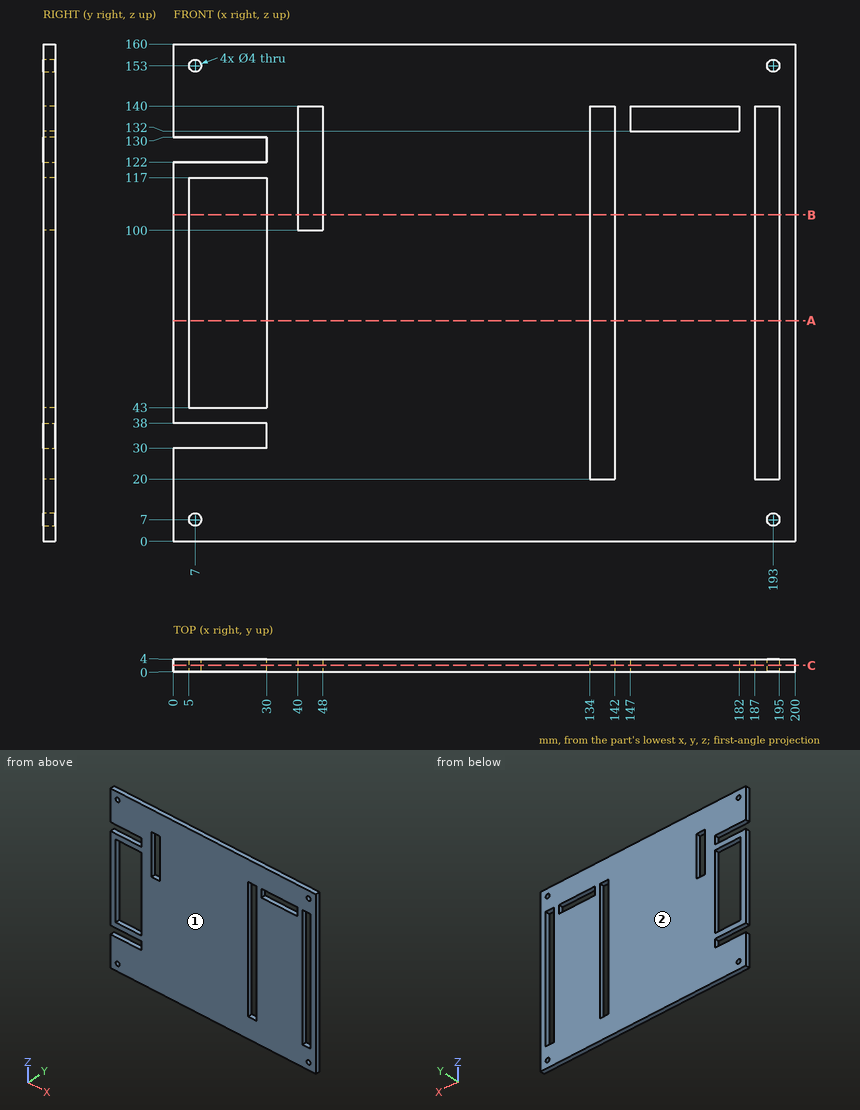
Source: three-view drawing plus pictorial views. Frame: mm from the lowest corner of the part. Give positions to 0.01 mm unless a question says otherwise; leave off trailing zeros. Write each loop counter-clockwise with the first axis right and the second up, starting at its lowest first coordinate (ties: lowest second). Pieces come first, ordered by that corner, then holes. Notation, with made-up numbers: (9.5, 61.25) - (30.5, 61.25) arc R16 cw to (30.5, 85.25) - close; hole circle Ø11 at (89.25, 30.25). An arc over 180 degrees is marked (long way). Write item = value, one per line. Start each with the question number.
Q1. Cut plane A-A, the plane z = 71. Return loops of the section in (x, y).
Q2. Cut plane B-B, the plane z = 105. Return loops of the section in (x, y).
Q3. Material intervals for probe 1 along X at (y, z) = (1, 45.5); probe 2 along X at (y, z) = (2.5, 121); probe 3 along X at (y, z) = (3.45, 36), sorted ascending.
Q4. Pin query (flat end, axial travel): pin 1 Ø2 at (y, z) = (2, 124) entering from -X. Return the tip coordinate at first contact, or that it passes through.
Q5. Cut plane C-C, the plane y = 2.05. Give the number of separate pieces and of enclosed holes in the cut face, then the cut area to 3 significant figures.
Q6. Draft query along Y for the marked faces 1 and 2. Return one class per face: +Y half, -Y half, draft (parallel to the pull), parting line (faces both ways), or undercut.
Computed values:
q1.outline = (0, 0) - (5, 0) - (5, 4) - (0, 4) - close; (30, 0) - (134, 0) - (134, 4) - (30, 4) - close; (142, 0) - (187, 0) - (187, 4) - (142, 4) - close; (195, 0) - (200, 0) - (200, 4) - (195, 4) - close
q2.outline = (0, 0) - (5, 0) - (5, 4) - (0, 4) - close; (30, 0) - (40, 0) - (40, 4) - (30, 4) - close; (48, 0) - (134, 0) - (134, 4) - (48, 4) - close; (142, 0) - (187, 0) - (187, 4) - (142, 4) - close; (195, 0) - (200, 0) - (200, 4) - (195, 4) - close
q3.probe_1 = 0 to 5, 30 to 134, 142 to 187, 195 to 200
q3.probe_2 = 0 to 40, 48 to 134, 142 to 187, 195 to 200
q3.probe_3 = 30 to 134, 142 to 187, 195 to 200
q4.pin_1 = 30
q5.separate_pieces = 1
q5.enclosed_holes = 9
q5.area = 27,100 mm²
q6.face_1 = -Y half
q6.face_2 = +Y half
